Autodesk Fusion 360 part; units mm, degrees
sketch "Sketch1" plane through (0, 0, 0) normal (0, 1, 0) x (1, 0, 0)
  circle A0 centre (0, 0) radius 63
  circle A1 centre (0, 0) radius 78
  circle A2 centre (0, 0) radius 22.5
  circle A3 centre (0, -70.5) radius 2.5
  circle A4 centre (61.0548, -35.25) radius 2.5
  circle A5 centre (61.0548, 35.25) radius 2.5
  circle A6 centre (0, 70.5) radius 2.5
  circle A7 centre (-61.0548, 35.25) radius 2.5
  circle A8 centre (-61.0548, -35.25) radius 2.5
  dimension "d1" = 126
  dimension "d2" = 15
  dimension "d3" = 45
  dimension "d14" = 5
  dimension "d15" = 70.5
  dimension "d17" = 360
extrude "Extrude1" add sketch "Sketch1" along normal blind 5 contours A1 | A3 | A4 | A5 | A6 | A7 | A8 makes body 1
move_face "OffsetFaces1" offset 65 1 faces at (62.9217, 3.3333, 3.1403) on bodies 1
extrude "Extrude2" add sketch "Sketch1" against normal blind 55 contours A2 bodies 1
sketch "Sketch3" plane through (0, -55, 0) normal (0, -1, 0) x (1, 0, 0)
  circle A0 centre (0, 0) radius 22.5
  circle A1 centre (0, 0) radius 37.5
  circle A2 centre (0, 32.5) radius 2.5
  circle A3 centre (-28.1458, 16.25) radius 2.5
  circle A4 centre (-28.1458, -16.25) radius 2.5
  circle A5 centre (0, -32.5) radius 2.5
  circle A6 centre (28.1458, -16.25) radius 2.5
  circle A7 centre (28.1458, 16.25) radius 2.5
  circle A8 centre (0, 0) radius 27.5
  dimension "d11" = 75
  dimension "d18" = 5
  dimension "d19" = 32.5
  dimension "d21" = 360
  dimension "d26" = 55
extrude "Extrude3" add sketch "Sketch3" against normal blind 5 contours A1 | A2 | A3 | A4 | A5 | A6 | A7 | A8 bodies 1
extrude "Extrude4" cut sketch "Sketch1" along normal blind 10 contours A3 | A4 | A5 | A6 | A7 | A8 bodies 1
extrude "Extrude5" cut sketch "Sketch3" against normal blind 10 contours A2 | A3 | A4 | A5 | A6 | A7 bodies 1
extrude "Extrude6" cut sketch "Sketch3" against normal blind 60 contours A0 bodies 1 makes body 2 at (40.4178, 0, -38.0861)
extrude "Extrude7" add sketch "Sketch3" against normal blind 60 contours A8 bodies 1 2
CAD build for the part. Positions are in the model's coordinates, mm. A direction names the side the tool comes from. Round coordinates to 2 decimals unless told otherwise and drop trailing zeros. Write each loop counter-clockwise with the first axis right and the second up, starting at its lowest first coordinate (ties: lowest second). Pieces come first, ordered by that corner, then holes. Notation, with made-up numbers: M -27.75,84.25 L -5.75,84.25 A22 cw -5.75,92.25 Z; hole C 38.5,-2 d7. An arc over 180 degrees is marked long. Put each result on its own line as item: value. Start each with the question number.
1) Saw through at A-A, the plane z = 0. Write the cut outline in (x, y), and give its area (4 significant figures).
2) 3-axis set-ups, long thin cutter, end or side, ignore diameter. For faces 1 (the cylindrical face through (0, -53, -30)), 2 (the cylindrical face through (-0.54, 2.46, 68.06)): which of +Z, -Z, +X, -X, +Y, -Y reach the whole face in a straight line?
3) Saw through at D-D, the plane y = -30.5. Write the cut outline in (x, z).
4) Drill centre lines: probe 1 along Z at (x, y) = (0, 3.25); probe 2 along X at (y, z) = (3.4, 35.25); probe 3 along X at (y, z) = (-23.5, 0.5). Where is each one in solid material? Low to high. Write a range as [from, to].
5) Pin check, flat tips, straight feed: pin 1 Ø1.5 at (x, y) = (-8.5, -7.5) entering from +Z; pin 2 Ø3 at (x, z) = (28.15, -16.25) entering from -Y; pin 3 Ø3 at (x, y) = (9, -17) entering from +Z; pin 4 Ø6.5 at (x, z) = (0, 32.5) entering from -Y. Stop position of each tip, or through.
6) Pull direction Z, two halves, no side cores. Call faces 3 (the cylindrical face through (-5.961, -25.35, -26.846)), 4 (the cylindrical face through (58.557, 2.465, -35.14)), 5 (the flat face through (-17, -50, -22)): pulls with the +Z half, pulls with the -Z half, needs draft (parallel to the pull), parting line crosses it, or undercut.
7) Saw through at B-B, the plane x = 0. Count the separate pieces of the cut face and the enclosed holes in it, and give its area (4 significant figures).
8) Saw through at C-C, the plane z = -16.25. Write the cut outline in (x, y).
Resolved:
1. outline: M -78,0 L -27.5,0 L -27.5,-50 L -37.5,-50 L -37.5,-55 L -22.5,-55 L -22.5,5 L -78,5 Z; M 22.5,-55 L 37.5,-55 L 37.5,-50 L 27.5,-50 L 27.5,0 L 78,0 L 78,5 L 22.5,5 Z
1. area: 1,205 mm²
2. face 1: -Y
2. face 2: +Y, -Y
3. outline: C 0,0 d55; hole C 0,0 d45
4. probe 1: [-78, -73], [-68, -22.5], [22.5, 68], [73, 78]
4. probe 2: [-69.58, -63.55], [-58.55, 58.55], [63.55, 69.58]
4. probe 3: [-27.5, -22.49], [22.49, 27.5]
5. pin 1: z = 26.39
5. pin 2: y = 0
5. pin 3: z = 26.46
5. pin 4: y = -55
6. face 3: parting line crosses it
6. face 4: undercut
6. face 5: needs draft
7. separate pieces: 6
7. enclosed holes: 0
7. area: 1,105 mm²
8. outline: M -76.29,0 L -22.19,0 L -22.19,-50 L -25.65,-50 L -25.65,-55 L -15.56,-55 L -15.56,5 L -76.29,5 Z; M -33.8,-55 L -30.65,-55 L -30.65,-50 L -33.8,-50 Z; M 15.56,-55 L 25.65,-55 L 25.65,-50 L 22.19,-50 L 22.19,0 L 76.29,0 L 76.29,5 L 15.56,5 Z; M 30.65,-55 L 33.8,-55 L 33.8,-50 L 30.65,-50 Z
